Autodesk Inventor part; units mm, degrees
ref_plane "Start Plane" through (0, 0, 5.2194) normal (0, 0, 1) x (1, 0, 0)
ref_plane "End Plane" through (0, 0, 330.8397) normal (0, 0, 1) x (1, 0, 0)
ref_plane "Work Plane4" through (9, 478.7803, -1071.6808) normal (0, 0.9444582, 0.3286315) x (1, 0, 0)
ref_plane "Start Plane" through (0, 0, 5.2194) normal (0, 0, 1) x (1, 0, 0)
ref_plane "End Plane" through (0, 0, 330.8397) normal (0, 0, 1) x (1, 0, 0)
sketch "Sketch" plane through (0, 0, 0) normal (0, 0, 1) x (1, 0, 0)
  line L0 (-15, -9) -> (-15, 9)
  line L1 (-9, 15) -> (9, 15)
  line L2 (15, 9) -> (15, -9)
  line L3 (9, -15) -> (-9, -15)
  arc A0 (-15, -9) -> (-9, -15) centre (-9, -9) ccw
  arc A1 (-9, 15) -> (-15, 9) centre (-9, 9) ccw
  arc A2 (15, 9) -> (9, 15) centre (9, 9) ccw
  arc A3 (9, -15) -> (15, -9) centre (9, -9) ccw
  arc A4 (-9, 12) -> (-12, 9) centre (-9, 9) ccw
  line L4 (-9, 12) -> (9, 12)
  arc A5 (12, 9) -> (9, 12) centre (9, 9) ccw
  line L5 (12, 9) -> (12, -9)
  arc A6 (9, -12) -> (12, -9) centre (9, -9) ccw
  line L6 (9, -12) -> (-9, -12)
  arc A7 (-12, -9) -> (-9, -12) centre (-9, -9) ccw
  line L7 (-12, -9) -> (-12, 9)
  line L8 (0, 22.7397) -> (0, -22.7397) construction
  line L9 (-22.7397, 0) -> (22.7397, 0) construction
  dimension "d7" = 6
  dimension "d10" = 30
  dimension "d11" = 30
  dimension "d12" = 3
  dimension "d15" = 15
  dimension "d16" = 15
extrude "Body" add sketch "Sketch" along normal up to surface (325.6204 mm away) from surface at 5.2194
sketch "Sketch3" plane through (0, 0, 0) normal (0, 0, 1) x (1, 0, 0)
  line L0 (0, 0) -> (10, 0)
ref_plane "Work Plane3" through (0, 0, 0) normal (0, -1, 0) x (1, 0, 0)
ref_plane "Work Plane4" through (9, 478.7803, -1071.6808) normal (0, 0.9444582, 0.3286315) x (1, 0, 0)
split "Split1" plane through (9, 478.7803, -1071.6808) removes the side toward (0, 0.9444582, 0.3286315)
ref_plane "Work Plane5" through (9, -205.4654, 283.6622) normal (0, -0.7840027, -0.6207574) x (1, 0, 0)
split "Split2" plane through (9, -205.4654, 283.6622) removes the side toward (0, -0.7840027, -0.6207574)
ref_plane "Work Plane6" through (9, 4.9295, 335.7692) normal (0, -0.3286315, 0.9444582) x (1, 0, 0)
split "Split3" plane through (9, 4.9295, 335.7692) removes the side toward (0, -0.3286315, 0.9444582)
sketch "Sketch4" plane through (0, 0, 0) normal (0, -1, 0) x (1, 0, 0)
  line L0 (-2, 5.2194) -> (12, 5.2194)
  line L1 (-2, 330.8397) -> (12, 330.8397)
  dimension "d18" = 325.6204
equation "\"d7\" = G_IR"
equation "\"d10\" = G_H"
equation "\"d11\" = G_W"
equation "\"d12\" = G_T"
equation "\"d15\" = 0.5 * d10"
equation "\"d16\" = 0.5 * d11"
equation "\"d3\" = G_L"
equation "\"G_W\" = 30"
equation "\"G_H\" = 30"
equation "\"G_T\" = 3"
equation "\"G_IR\" = 6"
equation "\"G_L\" = d18"
equation "\"G_OFFSET_START\" = -5.21936"
equation "\"G_OFFSET_END\" = -19.09635"
equation "\"d13\" = -G_OFFSET_START"
equation "\"d14\" = G_OFFSET_END + B_L"
equation "\"B_L\" = 349.93607"
properties part number "DIN EN 10219-2 - 30 x 30 x 3  - 325.62" material "Steel, Mild"
Read the model definition and answer for the solid it produces. Units are mm, in the model's axes. A direction names the side the tool comes from. Round coordinates to 2 decimals unless told otherwise and drop trailing zeros. Write each loop counter-clockwise with the first axis right and the second up, starting at its lowest first coordinate (ties: lowest second). Pieces come first, ordered by that corner, then holes.
1. Which of the six approach directions +Z, -Z, +X, -X, +Y, -Y give full straight-line access (tool end or side, diameter ignored) to faces 5 (the face through (15, 0, 169)), 6 (the face through (12, 0, 169))?
2. The part is cut by section A-A, the plane x = 4. Determine the outline of the cut face in (y, z).
3. The part is cut by section B-B, the plane z = 216.5. Determine the outline of the cut face in (x, y), then the cut area to 3 significant figures.
4. The part is cut by section C-C, the plane y = -5. Determine the outline of the cut face in (x, z).
5. Straight lines are drawn through the part: L1, parallel to X at y = -3.5, z = 91; L2, parallel to Y at x = -11, z = 188. For each, find the intervals that lie inside material, in ascending order.
6. Determine the mould class of faces 1 (the face through (-13.196, -13.289, 181.118)), 2 (the face through (13.196, 13.289, 139.911)), 3 (the face through (0, 12, 138)), 4 (the face through (0, -12, 183)) for opening direction Y: pulls with the +Y half, pulls with the -Y half, needs draft (parallel to the pull), parting line crosses it, or undercut.
7. Given pin 1 Ø2 at (x, y) = (11.5, -3.5) entering from -Z; pin 2 Ø1.5 at (x, z) = (10.5, 91.5) entering from +Y; pin 3 Ø1.5 at (y, z) = (-10.5, 108.5) entering from +X; pin 4 Ø8 at (y, z) = (-10, 186) entering from -X, each flat-ended and moving along its own axis, determine where each tip first touches the part or whether it passes through.
Values:
1. face 5: +Z, -Z, +X, +Y, -Y
1. face 6: +Z, -Z
2. outline: (-15, 43.11) - (-12, 39.32) - (-12, 329.88) - (-15, 328.83) - close; (12, 9.01) - (15, 5.22) - (15, 261.18) - (12, 269.8) - close
3. outline: (-15, -9) arc R6 ccw to (-9, -15) - (9, -15) arc R6 ccw to (15, -9) - (15, 9) arc R6 ccw to (9, 15) - (-9, 15) arc R6 ccw to (-15, 9) - close; hole (-12, -9) arc R3 ccw to (-9, -12) - (9, -12) arc R3 ccw to (12, -9) - (12, 9) arc R3 ccw to (9, 12) - (-9, 12) arc R3 ccw to (-12, 9) - close
3. area: 301 mm2
4. outline: (-15, 30.48) - (-12, 30.48) - (-12, 318.66) - (-15, 318.66) - close; (12, 30.48) - (15, 30.48) - (15, 318.66) - (12, 318.66) - close
5. L1: x = -15 to -12, 12 to 15
5. L2: y = -14.66 to -11.24, 11.24 to 14.66
6. face 1: pulls with the -Y half
6. face 2: pulls with the +Y half
6. face 3: undercut
6. face 4: undercut
7. pin 1: stops at z = 27.49
7. pin 2: stops at y = 14.95
7. pin 3: stops at x = 14.95
7. pin 4: stops at x = -15
